Design review of the part built by this model. Coordinates are the model's own, in mm. Face numbers are marked on the shaded views. Give positions to 0.01 mm unless a question says otherwise; leave off trailing zeros. Write each loop counter-clockwise with the first axis right and the second up, starting at its lowest first coordinate (ties: lowest second). Pieces come first, ordered by that corner, then holes. Notation, with made-up numbers: (35, 84.5) -> (59, 84.5) arc R24 ccw to (59, 122.5) -> close; hole circle Ø6 at (0, 44). An arc over 180 degrees is marked (long way). Use CSV: the item, a comma, the result in double quotes.
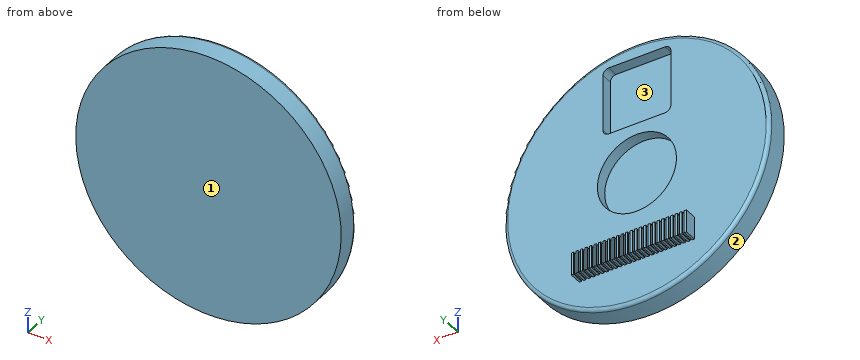
```python
from build123d import *

# Parameters (mm, degrees)
SKETCH1_R           = 117.5
BOSS_EXTRUDE1_DEPTH = 20
SKETCH2_R           = 35
CUT_EXTRUDE1_DEPTH  = 10
SKETCH3_W           = 102
SKETCH3_H           = 20
BOSS_EXTRUDE2_DEPTH = 10
SKETCH6_W           = 2
SKETCH6_H           = 20
BOSS_EXTRUDE3_DEPTH = 1
SKETCH7_W           = 2
SKETCH7_H           = 10
CUT_EXTRUDE2_DEPTH  = 1
SKETCH8_W           = 2
SKETCH8_H           = 10
CUT_EXTRUDE3_DEPTH  = 1
FILLET3_R           = 3


with BuildPart() as part:
    # Sketch1 → Boss-Extrude1 (new body)
    with BuildSketch(Plane(origin=(0, 0, 0), x_dir=(1, 0, 0), z_dir=(0, 1, 0))):
        with Locations(Location((0, 0, 0), (0, 0, 270))):
            Circle(SKETCH1_R)
    extrude(amount=BOSS_EXTRUDE1_DEPTH)

    # Sketch2 → Cut-Extrude1 (cut)
    with BuildSketch(Plane(origin=(0, 20, 0), x_dir=(1, 0, 0), z_dir=(0, 1, 0))):
        with Locations(Location((0, 0, 0), (0, 0, 270))):
            Circle(SKETCH2_R)
        with BuildLine():
            Line((-25, -105), (25, -105))
            ThreePointArc((25, -105), (28.535533906, -103.535533906), (30, -100))
            Line((30, -100), (30, -50))
            ThreePointArc((30, -50), (28.535533906, -46.464466094), (25, -45))
            Line((25, -45), (-25, -45))
            ThreePointArc((-25, -45), (-28.535533906, -46.464466094), (-30, -50))
            Line((-30, -50), (-30, -100))
            ThreePointArc((-30, -100), (-28.535533906, -103.535533906), (-25, -105))
        make_face()
    extrude(amount=-CUT_EXTRUDE1_DEPTH, mode=Mode.SUBTRACT)

    # Sketch3 → Boss-Extrude2 (add)
    with BuildSketch(Plane(origin=(0, 20, 0), x_dir=(1, 0, 0), z_dir=(0, 1, 0))):
        with Locations((0, 70)):
            Rectangle(SKETCH3_W, SKETCH3_H)
    extrude(amount=BOSS_EXTRUDE2_DEPTH)

    # Sketch6 → Boss-Extrude3 (add)
    with BuildSketch(Plane(origin=(0, 30, 0), x_dir=(1, 0, 0), z_dir=(0, 1, 0))):
        with Locations((-50, 70)):
            Rectangle(SKETCH6_W, SKETCH6_H)
        with Locations((-46, 70)):
            Rectangle(SKETCH6_W, SKETCH6_H)
        with Locations((-42, 70)):
            Rectangle(SKETCH6_W, SKETCH6_H)
        with Locations((-38, 70)):
            Rectangle(SKETCH6_W, SKETCH6_H)
        with Locations((-34, 70)):
            Rectangle(SKETCH6_W, SKETCH6_H)
        with Locations((-30, 70)):
            Rectangle(SKETCH6_W, SKETCH6_H)
        with Locations((-26, 70)):
            Rectangle(SKETCH6_W, SKETCH6_H)
        with Locations((-22, 70)):
            Rectangle(SKETCH6_W, SKETCH6_H)
        with Locations((-18, 70)):
            Rectangle(SKETCH6_W, SKETCH6_H)
        with Locations((-14, 70)):
            Rectangle(SKETCH6_W, SKETCH6_H)
        with Locations((-10, 70)):
            Rectangle(SKETCH6_W, SKETCH6_H)
        with Locations((-6, 70)):
            Rectangle(SKETCH6_W, SKETCH6_H)
        with Locations((-2, 70)):
            Rectangle(SKETCH6_W, SKETCH6_H)
        with Locations((2, 70)):
            Rectangle(SKETCH6_W, SKETCH6_H)
        with Locations((6, 70)):
            Rectangle(SKETCH6_W, SKETCH6_H)
        with Locations((10, 70)):
            Rectangle(SKETCH6_W, SKETCH6_H)
        with Locations((14, 70)):
            Rectangle(SKETCH6_W, SKETCH6_H)
        with Locations((18, 70)):
            Rectangle(SKETCH6_W, SKETCH6_H)
        with Locations((22, 70)):
            Rectangle(SKETCH6_W, SKETCH6_H)
        with Locations((26, 70)):
            Rectangle(SKETCH6_W, SKETCH6_H)
        with Locations((30, 70)):
            Rectangle(SKETCH6_W, SKETCH6_H)
        with Locations((34, 70)):
            Rectangle(SKETCH6_W, SKETCH6_H)
        with Locations((38, 70)):
            Rectangle(SKETCH6_W, SKETCH6_H)
        with Locations((42, 70)):
            Rectangle(SKETCH6_W, SKETCH6_H)
        with Locations((46, 70)):
            Rectangle(SKETCH6_W, SKETCH6_H)
        with Locations((50, 70)):
            Rectangle(SKETCH6_W, SKETCH6_H)
    extrude(amount=BOSS_EXTRUDE3_DEPTH)

    # Sketch7 → Cut-Extrude2 (cut)
    with BuildSketch(Plane.XY.offset(-60)):
        with Locations((-48, 25)):
            Rectangle(SKETCH7_W, SKETCH7_H)
        with Locations((-44, 25)):
            Rectangle(SKETCH7_W, SKETCH7_H)
        with Locations((-40, 25)):
            Rectangle(SKETCH7_W, SKETCH7_H)
        with Locations((-36, 25)):
            Rectangle(SKETCH7_W, SKETCH7_H)
        with Locations((-32, 25)):
            Rectangle(SKETCH7_W, SKETCH7_H)
        with Locations((-28, 25)):
            Rectangle(SKETCH7_W, SKETCH7_H)
        with Locations((-24, 25)):
            Rectangle(SKETCH7_W, SKETCH7_H)
        with Locations((-20, 25)):
            Rectangle(SKETCH7_W, SKETCH7_H)
        with Locations((-16, 25)):
            Rectangle(SKETCH7_W, SKETCH7_H)
        with Locations((-12, 25)):
            Rectangle(SKETCH7_W, SKETCH7_H)
        with Locations((-8, 25)):
            Rectangle(SKETCH7_W, SKETCH7_H)
        with Locations((-4, 25)):
            Rectangle(SKETCH7_W, SKETCH7_H)
        with Locations((0, 25)):
            Rectangle(SKETCH7_W, SKETCH7_H)
        with Locations((4, 25)):
            Rectangle(SKETCH7_W, SKETCH7_H)
        with Locations((8, 25)):
            Rectangle(SKETCH7_W, SKETCH7_H)
        with Locations((12, 25)):
            Rectangle(SKETCH7_W, SKETCH7_H)
        with Locations((16, 25)):
            Rectangle(SKETCH7_W, SKETCH7_H)
        with Locations((20, 25)):
            Rectangle(SKETCH7_W, SKETCH7_H)
        with Locations((24, 25)):
            Rectangle(SKETCH7_W, SKETCH7_H)
        with Locations((28, 25)):
            Rectangle(SKETCH7_W, SKETCH7_H)
        with Locations((32, 25)):
            Rectangle(SKETCH7_W, SKETCH7_H)
        with Locations((36, 25)):
            Rectangle(SKETCH7_W, SKETCH7_H)
        with Locations((40, 25)):
            Rectangle(SKETCH7_W, SKETCH7_H)
        with Locations((44, 25)):
            Rectangle(SKETCH7_W, SKETCH7_H)
        with Locations((48, 25)):
            Rectangle(SKETCH7_W, SKETCH7_H)
    extrude(amount=-CUT_EXTRUDE2_DEPTH, mode=Mode.SUBTRACT)

    # Sketch8 → Cut-Extrude3 (cut)
    with BuildSketch(Plane(origin=(0, 0, -80), x_dir=(-1, 0, 0), z_dir=(0, 0, -1))):
        with Locations((-48, 25)):
            Rectangle(SKETCH8_W, SKETCH8_H)
        with Locations((-44, 25)):
            Rectangle(SKETCH8_W, SKETCH8_H)
        with Locations((-40, 25)):
            Rectangle(SKETCH8_W, SKETCH8_H)
        with Locations((-36, 25)):
            Rectangle(SKETCH8_W, SKETCH8_H)
        with Locations((-32, 25)):
            Rectangle(SKETCH8_W, SKETCH8_H)
        with Locations((-28, 25)):
            Rectangle(SKETCH8_W, SKETCH8_H)
        with Locations((-24, 25)):
            Rectangle(SKETCH8_W, SKETCH8_H)
        with Locations((-20, 25)):
            Rectangle(SKETCH8_W, SKETCH8_H)
        with Locations((-16, 25)):
            Rectangle(SKETCH8_W, SKETCH8_H)
        with Locations((-12, 25)):
            Rectangle(SKETCH8_W, SKETCH8_H)
        with Locations((-8, 25)):
            Rectangle(SKETCH8_W, SKETCH8_H)
        with Locations((-4, 25)):
            Rectangle(SKETCH8_W, SKETCH8_H)
        with Locations((0, 25)):
            Rectangle(SKETCH8_W, SKETCH8_H)
        with Locations((4, 25)):
            Rectangle(SKETCH8_W, SKETCH8_H)
        with Locations((8, 25)):
            Rectangle(SKETCH8_W, SKETCH8_H)
        with Locations((12, 25)):
            Rectangle(SKETCH8_W, SKETCH8_H)
        with Locations((16, 25)):
            Rectangle(SKETCH8_W, SKETCH8_H)
        with Locations((20, 25)):
            Rectangle(SKETCH8_W, SKETCH8_H)
        with Locations((24, 25)):
            Rectangle(SKETCH8_W, SKETCH8_H)
        with Locations((28, 25)):
            Rectangle(SKETCH8_W, SKETCH8_H)
        with Locations((32, 25)):
            Rectangle(SKETCH8_W, SKETCH8_H)
        with Locations((36, 25)):
            Rectangle(SKETCH8_W, SKETCH8_H)
        with Locations((40, 25)):
            Rectangle(SKETCH8_W, SKETCH8_H)
        with Locations((44, 25)):
            Rectangle(SKETCH8_W, SKETCH8_H)
        with Locations((48, 25)):
            Rectangle(SKETCH8_W, SKETCH8_H)
    extrude(amount=-CUT_EXTRUDE3_DEPTH, mode=Mode.SUBTRACT)

    # Fillet3
    fillet3_edges = [part.edges().sort_by_distance(p)[0] for p in [
        (0, 20, -117.5),
    ]]
    fillet(fillet3_edges, radius=FILLET3_R)


solid = part.part
```
(1) Clearance check with flat-ended pins moving along their axes: pin 1 (3.5 mm diameter, centred on y = 24, z = -65.5, fed in from -X); pin 2 (1 mm diameter, centred on x = 14, y = 25, fed in from +Z); pin 3 (6 mm diameter, centred on y = 19.5, z = -27, fed in from -X). State where each tip first meets the part, or that it passes through.
Established:
pin 1,"stops at x = -51"
pin 2,"stops at z = -60"
pin 3,"stops at x = -114.82"
(2) Take a section at B-B (z = 0). Write out the cut boundary in (x, y), then the cut area to 3 significant figures.
Established:
outline,"(-117.5, 0) -> (117.5, 0) -> (117.5, 17) arc R3 ccw to (114.5, 20) -> (35, 20) -> (35, 10) -> (-35, 10) -> (-35, 20) -> (-114.5, 20) arc R3 ccw to (-117.5, 17) -> close"
area,"4,000 mm2"
(3) For line 1 along X through (y, z) = (16, 0); line 2 along Y through (x, z) = (40.5, -34.5); line 3 along X through (y, z) = (18, 0), list the stretches that pass through material, from the lowest coordinate up. Write a range as [from, to].
Established:
line 1,"x = [-117.5, -35], [35, 117.5]"
line 2,"y = [0, 20]"
line 3,"x = [-117.33, -35], [35, 117.33]"
(4) Take a section at A-A (y = 13.5). Write out the cut boundary in (x, z).
Established:
outline,"circle Ø235 at (0, 0); hole circle Ø70 at (0, 0); hole (-30, 50) arc R5 ccw to (-25, 45) -> (25, 45) arc R5 ccw to (30, 50) -> (30, 100) arc R5 ccw to (25, 105) -> (-25, 105) arc R5 ccw to (-30, 100) -> close"
(5) Mouldability with a two-part tool opening along X and no side actions: class the marked faces 1, 2 and 3 as +X half, -X half, draft (parallel to the pull), parting line (faces both ways), or undercut.
Established:
face 1,"draft"
face 2,"parting line"
face 3,"undercut"
